Design review of the part shown in the three views and the two pictorial views. Dimensions are in mm from the part's minimum x, y and z. A direction names the side the tool comes from. Give positions to 0.01 mm unless a question says otherwise; leave off trailing zeros. Write each loop counter-clockwise with the first axis right and the second up, starting at its lowest first coordinate (ties: lowest second). Pieces come first, ordered by that corner, then holes. Notation, with made-up numbers: (66, 10.5) -> (87, 10.5) arc R17 ccw to (87, 37.5) -> close; hole circle Ø8 at (76.25, -0.5). An arc over 180 degrees is marked (long way). Return JSON: item names as keys, results as strings. Group by question number.
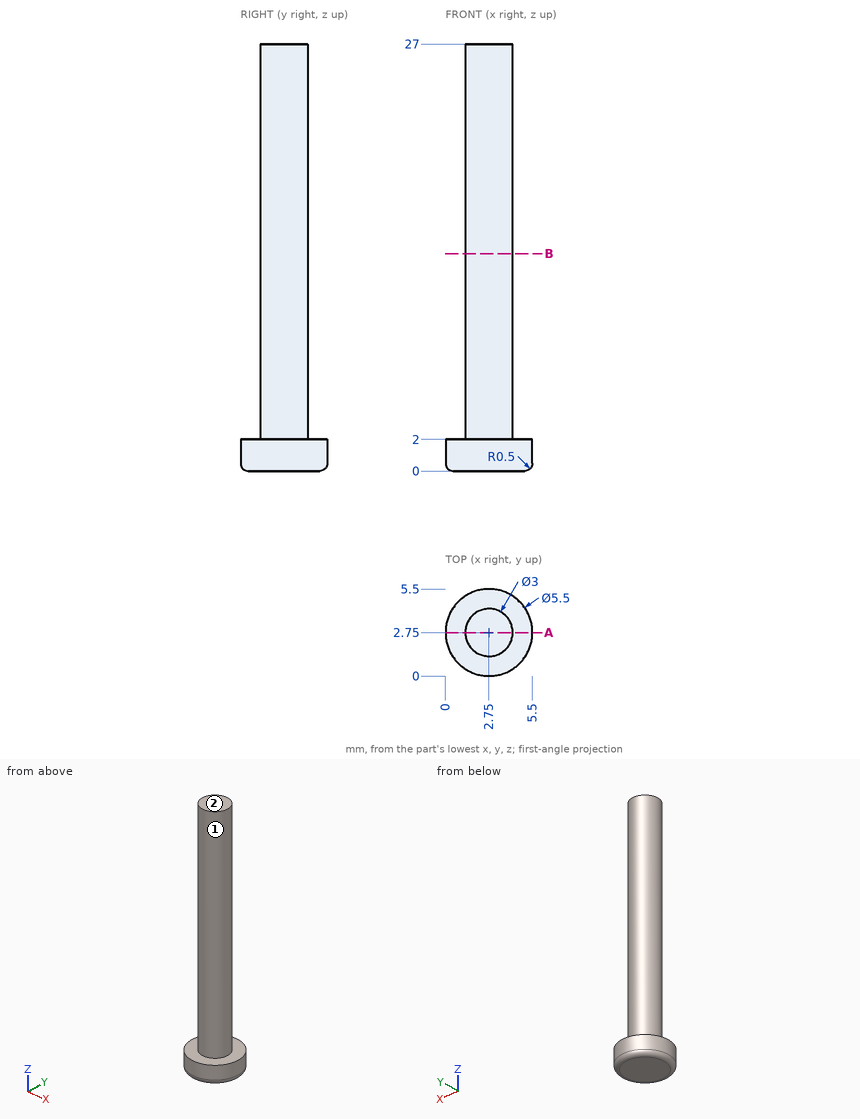
Q1. Take a section at A-A, the plane y = 2.75. Give the boundary of the cut face in (x, z).
Q2. Insertion check: pin 1 (1.5 mm diameter, centred on y = 3, z = 3.5, fed in from -X); pin 2 (2 mm diameter, centred on x = 4, z = 14, fed in from +Y). Each pin has a flat end and moves straight along its axis. Give the tip position at first contact, or say it passes through.
Q3. For L1, parallel to Y at x = 2.7, z = 17.5; L2, parallel to Z at x = 2.95, y = 0.85; L3, parallel to X at y = 3.75, z = 5.75, list the stretches that pass through material, from the lowest coordinate up. Write a range as from..to.
Q4. Take a section at B-B, the plane z = 13.75. Give the boundary of the cut face in (x, y).
Q5. Tool access review of the marked faces 1 and 2: name each direction out of +Z, -Z, +X, -X, +Y, -Y from which nothing blocks a thin tool from reaching the whole face with its end or side.
Final values:
{
 "1": {"outline": "(0, 0.5) arc R0.5 ccw to (0.5, 0) -> (5, 0) arc R0.5 ccw to (5.5, 0.5) -> (5.5, 2) -> (4.25, 2) -> (4.25, 27) -> (1.25, 27) -> (1.25, 2) -> (0, 2) -> close"},
 "2": {"pin 1": "stops at x = 1.25", "pin 2": "stops at y = 4.23"},
 "3": {"L1": "y = 1.25..4.25", "L2": "z = 0..2", "L3": "x = 1.63..3.87"},
 "4": {"outline": "circle Ø3 at (2.75, 2.75)"},
 "5": {"face 1": "+Z", "face 2": "+Z, +X, -X, +Y, -Y"}
}
